Geometry: final body of the model. Coordinates: model frame, mm. A direction names the side the tool comes from. Coordinates: 2 decimals unless noted, no trailing zeros. Order: outer loops, then holes, each group sorted by start corner. A loop starts at its lowest first (then second) coordinate and runs counter-clockwise, first axis right, second up. Notation, with made-up numbers: M -3,4.25 L 23,4.25 A21 cw 23,25.25 Z; hole C 76,16 d3. An arc over 180 degrees is marked long. Use CSV: the item, a comma, the result in double quotes. Start each with the question number.
Q1. Ray query, probe 1 along Y at (x, z) = (-0.25, 2.5); probe 2 along X at (y, z) = (5.5, 5.5); probe 3 along X at (y, z) = (6, 2.5). Return the intervals inside material, ascending.
Q2. Mould query, pull axis Y, two halves, no side actions, for faces 1 (the face through (5, -5, 0)), 2 (the face through (-13.297, -0.585, 3.138)), 3 (the face through (-1, -6.512, 3)). Classes: +Y half, -Y half, draft (parallel to the pull), parting line (faces both ways), or undercut.
Q3. First-contact query: P1, Ø3, axis at x = 8, z = 4.5, coming from the -Y side; P2, Ø1.5, axis at x = -4.5, y = -9.5, coming from the -Z side; P3, Ø2, axis at y = -6.5, z = 2.5, coming from the -X side; P4, Ø1, axis at y = -5.5, z = 3.5, coming from the -X side. Flat tips, straight axial feed; report the tip coordinate or a pass-through.
Q4. Access query for faces 4 (the face through (9, 0.6, 3)), 5 (the face through (5.06, -3.67, 0.26)), 6 (the face through (-1, 6.442, 3)), 7 (the face through (5.008, 3.69, 6.092)). Directions: +Z, -Z, +X, -X, +Y, -Y. A direction counts if a zero-diameter tool reaches every point of the face in a straight line with its end or side. Return the directions, or none.
Q5. Section query A-A, the plane z = 3.5. Output: boundary loops of the cut face in (x, y) (3 decimals).
Autodesk Inventor part; units mm, degrees
ref_plane "YZ Plane" through (0, 0, 0) normal (1, 0, 0) x (0, 1, 0)
ref_plane "XZ Plane" through (0, 0, 0) normal (0, 1, 0) x (-1, 0, 0)
ref_plane "XY Plane" through (0, 0, 0) normal (0, 0, 1) x (1, 0, 0)
sketch "Sketch1" plane through (0, 0, 0) normal (0, 0, 1) x (1, 0, 0)
  line L0 (-4.3488, 6.4416) -> (3.1302, 6.4416)
  line L1 (3.1302, 6.4416) -> (6.503, 0.5996)
  line L2 (6.503, -0.6704) -> (3.1302, -6.5124)
  line L3 (3.1302, -6.5124) -> (-4.3488, -6.5124)
  line L4 (-4.3488, -6.5124) -> (-7.7708, -0.5853)
  line L5 (-7.7708, 0.5145) -> (-4.3488, 6.4416)
  arc A0 (12.0748, 0.5996) -> (12.0748, -0.6704) centre (-0.6093, -0.0354) ccw
  arc A1 (-8.0883, 0.5996) -> (-8.0883, -0.6704) centre (-8.0883, -0.0354) ccw
  line L6 (-8.0883, 0.5996) -> (-7.7217, 0.5996)
  line L7 (6.503, 0.5996) -> (12.0748, 0.5996)
  line L8 (-8.0883, -0.6704) -> (-7.7217, -0.6704)
  line L9 (6.503, -0.6704) -> (12.0748, -0.6704)
  point P0 (-0.6093, 6.4416)
  dimension "d2" = 12.954
  dimension "d3" = 25.4
  dimension "d4" = 1.27
extrude "Extrusion1" add sketch "Sketch1" along normal blind 6.35
chamfer "Chamfer1" distance 0.508 angle 45 2 edges at (-13.3093, -0.0354, 6.35) (-13.3093, -0.0354, 0)
chamfer "Chamfer2" distance 0.508 angle 45 12 edges at (-6.0353, 3.5206, 6.35) (-0.6093, 6.4416, 6.35) (4.8166, 3.5206, 6.35) (4.8166, -3.5914, 6.35) (-0.6093, -6.5124, 6.35) (-6.0353, -3.5914, 6.35) (-6.0353, -3.5914, 0) (-6.0353, 3.5206, 0) (-0.6093, -6.5124, 0) (4.8166, -3.5914, 0) (4.8166, 3.5206, 0) (-0.6093, 6.4416, 0)
properties part number "Hex Shaft Collar"
Responses:
1,probe 1,"y = -12.73 to -6.51, 6.44 to 12.66"
1,probe 2,"x = -12.04 to -4.89, 3.67 to 10.82"
1,probe 3,"x = -11.78 to -4.6, 3.39 to 10.56"
2,face 1,"draft"
2,face 2,"parting line"
2,face 3,"undercut"
3,P1,"stops at y = -10.56"
3,P2,"stops at z = 0"
3,P3,"stops at x = -12.07"
3,P4,"stops at x = -12.3"
4,face 4,"+Z, -Z, +X"
4,face 5,"-Z"
4,face 6,"+Z, -Z"
4,face 7,"+Z"
5,outline,"M -8.088,-0.67 A0.635 cw -8.088,0.6 L -7.722,0.6 L -4.349,6.442 L 3.13,6.442 L 6.503,0.6 L 12.075,0.6 A12.7 ccw long 12.075,-0.67 L 6.503,-0.67 L 3.13,-6.512 L -4.349,-6.512 L -7.722,-0.67 Z"
